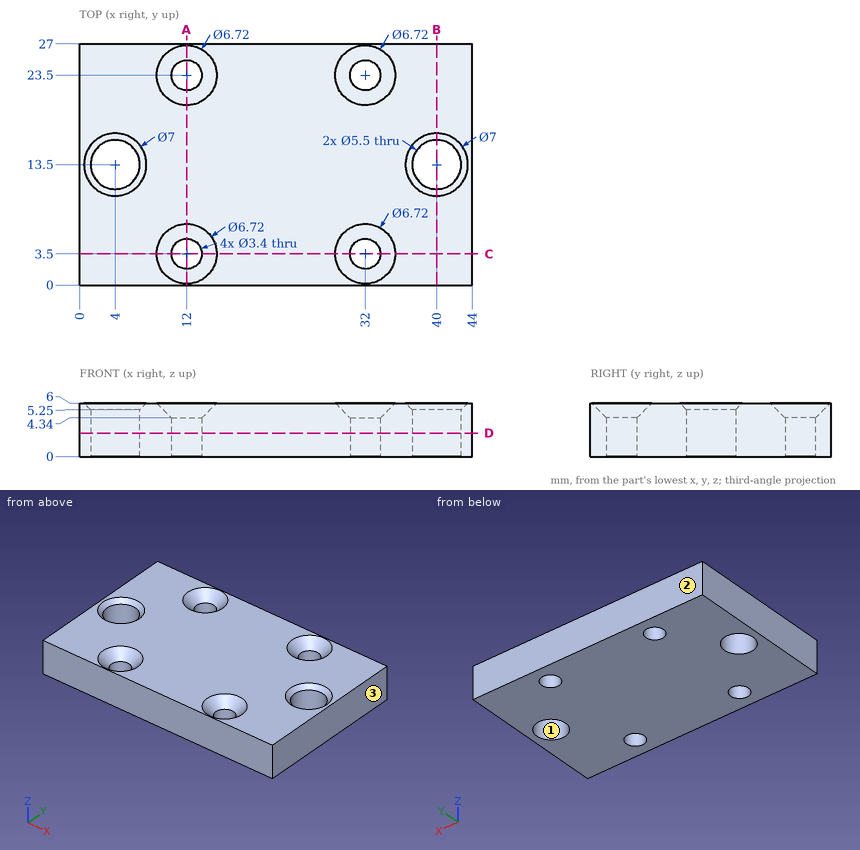
For this review, use the dimensioned drawing (mm, ordinates from the lowest corner) and the shaded views. Round coordinates to 2 decimals unless told otherwise and drop trailing zeros. Write each loop counter-clockwise with the first axis right and the second up, starting at its lowest first coordinate (ties: lowest second). Pieces come first, ordered by that corner, then holes. Notation, with made-up numbers: (8, 5) -> (60, 5) arc R17 ccw to (60, 25) -> close; hole circle Ø3 at (80, 49.25). An arc over 180 degrees is marked (long way). One line per item, written item: value. Start each with the question number.
Q1. Add section D-D (z = 2.65). Give the boundary of the cut face in (x, y), then the cut area to 3 significant figures.
Q2. Add section B-B (x = 40). Give the boundary of the cut face in (y, z), then the cut area to 3 significant figures.
Q3. Insertion check: P1, Ø5.5, axis at x = 12, y = 3.5, coming from the +Z side; P2, Ø2, axis at x = 32, y = 23.5, coming from the +Z side. Each pin has a flat end and moves straight along its axis. Give the tip position at first contact, or say it passes through.
Q4. The part is to be moulded in two halves that separate along X. For the marked faces 1, 2 and 3, say which applies: pulls with the +X half, pulls with the -X half, needs draft (parallel to the pull), parting line crosses it, or undercut.
Q5. To check wall thickness, follow probe 1 along Y at (x, z) = (32, 1.3); probe 2 along X at (y, z) = (23.5, 2.1); probe 3 along Y at (x, z) = (4, 2.2). State the ranges of each line that lie inside material, in increasing order.
Q6. Add section C-C (y = 3.5). Give the boundary of the cut face in (x, z), then the cut area to 3 significant figures.
Q7. Add section A-A (x = 12). Give the boundary of the cut face in (y, z), then the cut area to 3 significant figures.
Response:
1. outline: (0, 0) -> (44, 0) -> (44, 27) -> (0, 27) -> close; hole circle Ø5.5 at (4, 13.5); hole circle Ø3.4 at (12, 3.5); hole circle Ø3.4 at (12, 23.5); hole circle Ø3.4 at (32, 3.5); hole circle Ø3.4 at (32, 23.5); hole circle Ø5.5 at (40, 13.5)
1. area: 1,100 mm^2
2. outline: (0, 0) -> (10.75, 0) -> (10.75, 5.25) -> (10, 6) -> (0, 6) -> close; (16.25, 0) -> (27, 0) -> (27, 6) -> (17, 6) -> (16.25, 5.25) -> close
2. area: 128 mm^2
3. P1: stops at z = 5.39
3. P2: passes through
4. face 1: undercut
4. face 2: needs draft
4. face 3: pulls with the +X half
5. probe 1: y = 0 to 1.8, 5.2 to 21.8, 25.2 to 27
5. probe 2: x = 0 to 10.3, 13.7 to 30.3, 33.7 to 44
5. probe 3: y = 0 to 10.75, 16.25 to 27
6. outline: (0, 0) -> (10.3, 0) -> (10.3, 4.34) -> (8.64, 6) -> (0, 6) -> close; (13.7, 0) -> (30.3, 0) -> (30.3, 4.34) -> (28.64, 6) -> (15.36, 6) -> (13.7, 4.34) -> close; (33.7, 0) -> (44, 0) -> (44, 6) -> (35.36, 6) -> (33.7, 4.34) -> close
6. area: 218 mm^2
7. outline: (0, 0) -> (1.8, 0) -> (1.8, 4.34) -> (0.14, 6) -> (0, 6) -> close; (5.2, 0) -> (21.8, 0) -> (21.8, 4.34) -> (20.14, 6) -> (6.86, 6) -> (5.2, 4.34) -> close; (25.2, 0) -> (27, 0) -> (27, 6) -> (26.86, 6) -> (25.2, 4.34) -> close
7. area: 116 mm^2
